For this review, take the finished solid that the model builds, in its own axes (mm). A direction names the side the tool comes from. Round coordinates to 2 decimals unless told otherwise and drop trailing zeros. Order: outer loops, then holes, each group sorted by start corner. A loop starts at its lowest first (then second) coordinate and runs counter-clockwise, first axis right, second up. Notation, with made-up numbers: (48.5, 70) -> (101.5, 70) arc R27 ccw to (101.5, 109) -> close; hole circle Ø8 at (19, 67.5). An arc over 180 degrees is marked (long way). Use a Markdown table: item, result. Add a question column.
1) Draft analysis for pull direction Z (two halves, no side actions). For faces 1 (the face through (-27.8, -14.9, 2.5)), 2 (the face through (24.79, -32.04, -7.28)), 3 (the face through (-1, -15, 0)), 4 (the face through (-20.21, -32.04, -7.28)), state which applies: pulls with the +Z half, pulls with the -Z half, needs draft (parallel to the pull), parting line crosses it, or undercut.
2) Consider section A-A (y = -15). State the section outline as (x, z) points, plus the area to 3 significant figures.
3) Machinability: for faces 5 (the face through (-1, -29, -7)), 6 (the face through (-1, -35, -4)), which of the approach directions +Z, -Z, +X, -X, +Y, -Y give a long, thin tool a straight path to every point of the face, cutting with its end or side? Answer none if there is none.
4) Consider section D-D (z = -11.5). State the section outline as (x, y) points, plus the area to 3 significant figures.
5) Consider section B-B (x = -7). State the section outline as (y, z) points.
6) Clearance check with flat-ended pins moving along their axes: P1, Ø12, axis at x = -10.5, z = -7.5, coming from the +Y side; P2, Ø7.5, axis at x = 25, y = -15, coming from the -Z side; P3, Ø7.5, axis at x = -22.5, z = -8, coming from the -Y side; P4, Ø6.5, axis at x = -25, y = -15, coming from the +Z side. State where each tip first meets the part, or that it passes through.
7) Wall thickness on line 1 along X through (y, z) = (-31, -8.5); line 2 along Y through (x, z) = (-25, 3.95); line 3 along Z through (x, y) = (-22.5, -32.3): over which ranges is each line inside the solid? List them lowest first. Write a range as [from, to].
8) Consider section C-C (z = -8). State the section outline as (x, y) points, plus the area to 3 significant figures.
```python
from build123d import *

# Parameters (mm, degrees)
SKETCH_W        = 75
SKETCH_H        = 35
PAD_DEPTH       = 6
SKETCH001_W     = 75
SKETCH001_H     = 6
PAD001_DEPTH    = 15
SKETCH002_R     = 2.8
POCKET_DEPTH    = 21.001
SKETCH003_R     = 2.4
POCKET001_DEPTH = 35.001
FILLET_R        = 1
CHAMFER_SIZE    = 0.3
CHAMFER001_SIZE = 1
FILLET001_R     = 1
FILLET002_R     = 1


with BuildPart() as part:
    # Sketch → Pad (new body)
    with BuildSketch(Plane.XY):
        with Locations((0, -17.5)):
            Rectangle(SKETCH_W, SKETCH_H)
    extrude(amount=PAD_DEPTH)

    # Sketch001 (on Face5 of Pad) → Pad001 (join)
    with BuildSketch(Plane(origin=(0, 0, 0), x_dir=(1, 0, 0), z_dir=(0, 0, -1))):
        with Locations((0, 32)):
            Rectangle(SKETCH001_W, SKETCH001_H)
    extrude(amount=PAD001_DEPTH)

    # Sketch002 (on Face6 of Pad001) → Pocket (cut, through all)
    with BuildSketch(Plane.XY.offset(6)):
        with Locations((-25, -15)):
            Circle(SKETCH002_R)
        with Locations((25, -15)):
            Circle(SKETCH002_R)
    extrude(amount=-POCKET_DEPTH, mode=Mode.SUBTRACT)

    # Sketch003 (on Face8 of Pocket) → Pocket001 (cut, through all)
    with BuildSketch(Plane.XZ.offset(35)):
        with Locations((-22.5, -8)):
            Circle(SKETCH003_R)
        with Locations((22.5, -8)):
            Circle(SKETCH003_R)
    extrude(amount=-POCKET001_DEPTH, mode=Mode.SUBTRACT)

    # Fillet
    fillet_edges = [part.edges().sort_by_distance(p)[0] for p in [
        (-37.5, 0, 3),
        (-37.5, -35, -7.5),
        (37.5, -35, -7.5),
        (37.5, 0, 3),
        (37.5, -29, -7.5),
        (-37.5, -29, -7.5),
    ]]
    fillet(fillet_edges, radius=FILLET_R)

    # Chamfer
    chamfer_edges = [part.edges().sort_by_distance(p)[0] for p in [
        (-24.9, -29, -8),
        (20.1, -29, -8),
        (20.1, -35, -8),
        (-24.9, -35, -8),
    ]]
    chamfer(chamfer_edges, length=CHAMFER_SIZE)

    # Chamfer001
    chamfer001_edges = [part.edges().sort_by_distance(p)[0] for p in [
        (-37.5, -17.5, 6),
        (-37.207107, -34.707107, 6),
        (0, -35, 6),
        (37.207107, -34.707107, 6),
        (37.5, -17.5, 6),
        (37.207107, -0.292893, 6),
        (0, 0, 6),
        (-37.207107, -0.292893, 6),
        (-27.8, -15, 6),
        (22.2, -15, 6),
    ]]
    chamfer(chamfer001_edges, length=CHAMFER001_SIZE)

    # Fillet001
    fillet001_edges = [part.edges().sort_by_distance(p)[0] for p in [
        (0, 0, 0),
    ]]
    fillet(fillet001_edges, radius=FILLET001_R)

    # Fillet002
    fillet002_edges = [part.edges().sort_by_distance(p)[0] for p in [
        (-37.5, -32, -15),
        (-37.207107, -29.292893, -15),
        (0, -29, -15),
        (37.207107, -29.292893, -15),
        (37.5, -32, -15),
        (37.207107, -34.707107, -15),
        (0, -35, -15),
        (-37.207107, -34.707107, -15),
    ]]
    fillet(fillet002_edges, radius=FILLET002_R)


solid = part.part
```
Results list:
| question | item | result |
|---|---|---|
| 1 | face 1 | needs draft |
| 1 | face 2 | undercut |
| 1 | face 3 | pulls with the -Z half |
| 1 | face 4 | undercut |
| 2 | outline | (-37.5, 1) arc R1 ccw to (-36.5, 0) -> (-27.8, 0) -> (-27.8, 5) -> (-28.8, 6) -> (-36.5, 6) -> (-37.5, 5) -> close; (-22.2, 0) -> (22.2, 0) -> (22.2, 5) -> (21.2, 6) -> (-21.2, 6) -> (-22.2, 5) -> close; (27.8, 0) -> (36.5, 0) arc R1 ccw to (37.5, 1) -> (37.5, 5) -> (36.5, 6) -> (28.8, 6) -> (27.8, 5) -> close |
| 2 | area | 379 mm2 |
| 3 | face 5 | -Z, +X, -X, +Y |
| 3 | face 6 | +Z, -Z, +X, -X, -Y |
| 4 | outline | (-37.5, -34) arc R1 ccw to (-36.5, -35) -> (36.5, -35) arc R1 ccw to (37.5, -34) -> (37.5, -30) arc R1 ccw to (36.5, -29) -> (-36.5, -29) arc R1 ccw to (-37.5, -30) -> close |
| 4 | area | 449 mm2 |
| 5 | outline | (-35, -14) arc R1 ccw to (-34, -15) -> (-30, -15) arc R1 ccw to (-29, -14) -> (-29, 0) -> (-1, 0) arc R1 ccw to (0, 1) -> (0, 5) -> (-1, 6) -> (-34, 6) -> (-35, 5) -> close |
| 6 | P1 | y = -29 |
| 6 | P2 | z = 0 |
| 6 | P3 | y = -35 |
| 6 | P4 | z = 5.45 |
| 7 | line 1 | [-37.5, -24.85], [-20.15, 20.15], [24.85, 37.5] |
| 7 | line 2 | [-35, -17.8], [-12.2, 0] |
| 7 | line 3 | [-15, -10.4], [-5.6, 6] |
| 8 | outline | (-37.5, -34) arc R1 ccw to (-36.5, -35) -> (-25.2, -35) -> (-24.9, -34.7) -> (-24.9, -29.3) -> (-25.2, -29) -> (-36.5, -29) arc R1 ccw to (-37.5, -30) -> close; (-20.1, -34.7) -> (-19.8, -35) -> (19.8, -35) -> (20.1, -34.7) -> (20.1, -29.3) -> (19.8, -29) -> (-19.8, -29) -> (-20.1, -29.3) -> close; (24.9, -34.7) -> (25.2, -35) -> (36.5, -35) arc R1 ccw to (37.5, -34) -> (37.5, -30) arc R1 ccw to (36.5, -29) -> (25.2, -29) -> (24.9, -29.3) -> close |
| 8 | area | 391 mm2 |
